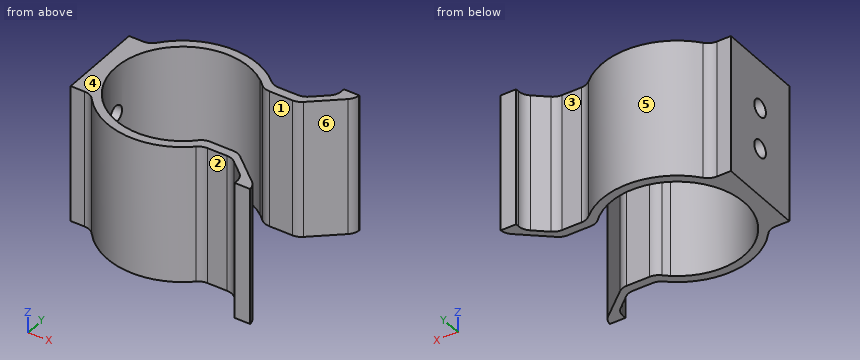
from build123d import *

# Parameters (mm, degrees)
F1_DEPTH = 50.8
F2_R     = 3.175
F3_DEPTH = 127
F5_DEPTH = 50.8
F6_DEPTH = 279.4
F7_R     = 5.08


with BuildPart() as f1:
    # F0 (on Top) → F1 (new body)
    with BuildSketch(Plane.XY):
        with BuildLine():
            ThreePointArc((20.2399183732, 19.2610826343), (21.625356316, 17.6914545532), (22.8893718502, 16.0224922001))
            Line((22.8893718502, 16.0224922001), (31.4840450883, 16.0224922001))
            Line((31.4840450883, 16.0224922001), (44.7927798103, 27.3874809633))
            Line((44.7927798103, 27.3874809633), (45.0897253182, 29.6793562902))
            Line((45.0897253182, 29.6793562902), (39.3924824893, 29.6793562902))
            Line((39.3924824893, 29.6793562902), (39.3924824893, 26.1115133762))
            Line((39.3924824893, 26.1115133762), (31.3704274416, 19.2610826343))
            Line((31.3704274416, 19.2610826343), (20.2399183732, 19.2610826343))
        make_face()
        with BuildLine():
            Line((31.4840450883, -16.0224922001), (22.8893718502, -16.0224922001))
            ThreePointArc((22.8893718502, -16.0224922001), (21.625356316, -17.6914545532), (20.2399183732, -19.2610826343))
            Line((20.2399183732, -19.2610826343), (31.3704274416, -19.2610826343))
            Line((31.3704274416, -19.2610826343), (39.3924824893, -26.1115133762))
            Line((39.3924824893, -26.1115133762), (39.3924824893, -29.6793562902))
            Line((39.3924824893, -29.6793562902), (45.0897253182, -29.6793562902))
            Line((45.0897253182, -29.6793562902), (44.7927798103, -27.3874809633))
            Line((44.7927798103, -27.3874809633), (31.4840450883, -16.0224922001))
        make_face()
        with BuildLine():
            ThreePointArc((15.5664999519, -19.2610826343), (-24.765, 0), (15.5664999519, 19.2610826343))
            Line((15.5664999519, 19.2610826343), (20.2399183732, 19.2610826343))
            ThreePointArc((20.2399183732, 19.2610826343), (-27.94, 0), (20.2399183732, -19.2610826343))
            Line((20.2399183732, -19.2610826343), (15.5664999519, -19.2610826343))
        make_face()
        with BuildLine():
            ThreePointArc((15.5664999519, 19.2610826343), (17.3009251144, 17.7195715294), (18.8834575408, 16.0224922001))
            Line((18.8834575408, 16.0224922001), (22.8893718502, 16.0224922001))
            ThreePointArc((22.8893718502, 16.0224922001), (21.625356316, 17.6914545532), (20.2399183732, 19.2610826343))
            Line((20.2399183732, 19.2610826343), (15.5664999519, 19.2610826343))
        make_face()
        with BuildLine():
            Line((22.8893718502, -16.0224922001), (18.8834575408, -16.0224922001))
            ThreePointArc((18.8834575408, -16.0224922001), (17.3009251144, -17.7195715294), (15.5664999519, -19.2610826343))
            Line((15.5664999519, -19.2610826343), (20.2399183732, -19.2610826343))
            ThreePointArc((20.2399183732, -19.2610826343), (21.625356316, -17.6914545532), (22.8893718502, -16.0224922001))
        make_face()
    extrude(amount=F1_DEPTH)

    # F2 (on Right) → F3 (cut)
    with BuildSketch(Plane.YZ):
        with Locations((0, 33.02)):
            Circle(F2_R)
        with Locations((0, 17.78)):
            Circle(F2_R)
    extrude(amount=-F3_DEPTH, mode=Mode.SUBTRACT)

    # F4 (on face) → F5 (join)
    with BuildSketch(Plane.XY.offset(50.8)):
        Polygon((-26.6156196594, 0), (-22.9919110776, 15.875), (-30.6119110776, 15.875), (-30.6119110776, -15.875), (-22.9919110776, -15.875), align=None)
    extrude(amount=-F5_DEPTH)

    # F2 (on Right) → F6 (cut)
    with BuildSketch(Plane.YZ):
        with Locations((0, 33.02)):
            Circle(F2_R)
        with Locations((0, 17.78)):
            Circle(F2_R)
    extrude(amount=-F6_DEPTH, mode=Mode.SUBTRACT)

    # F7
    f7_edges = [f1.edges().sort_by_distance(p)[0] for p in [
        (-22.991911, 15.875, 25.4),
        (-22.991911, -15.875, 25.4),
        (20.239918, -19.261083, 25.4),
        (31.370427, -19.261083, 25.4),
        (39.392482, -26.111513, 25.4),
        (31.484045, -16.022492, 25.4),
        (18.883458, -16.022492, 25.4),
        (44.79278, -27.387481, 25.4),
        (44.79278, 27.387481, 25.4),
        (31.484045, 16.022492, 25.4),
        (31.370427, 19.261083, 25.4),
        (39.392482, 26.111513, 25.4),
        (20.239918, 19.261083, 25.4),
        (18.883458, 16.022492, 25.4),
    ]]
    fillet(f7_edges, radius=F7_R)


solid = f1.part
Geometry check sheet. Reference: the model listing, model coordinates, mm. Face numbers are marked on the shaded views. A direction names the side the tool comes from. Give positions to 0.01 mm unless a question says otherwise; leave off trailing zeros. Write each loop counter-clockwise with the first axis right and the second up, starting at its lowest first coordinate (ties: lowest second). Pieces come first, ordered by that corner, then holes. Notation, with made-up numbers: M 58.5,-2.75 L 64.5,-2.75 A23 cw 64.5,20.25 Z; hole C 56.5,-24.75 d4. An arc over 180 degrees is marked long. One line per question, with ' | ' between items.
1. Scan lines: line 1 along Z through (x, y) = (-26, 0) (3 decimals); line 2 along Y through (x, z) = (0, 28) (3 decimals); line 3 along Y through (x, z) = (-28.5, 17.78) (3 decimals). Record each from-to range of solid material in increasing order. Write a range as from..to.
Ans:
line 1: 0..14.605, 20.955..29.845, 36.195..50.8 | line 2: -27.94..-24.765, 24.765..27.94 | line 3: -15.875..-3.175, 3.175..15.875
2. Cross-section at B-B (x = 0). Enter the section's corners in (y, z) (3 decimals), plus the area to 3 significant figures.
Ans:
outline: M -27.94,0 L -24.765,0 L -24.765,50.8 L -27.94,50.8 Z; M 24.765,0 L 27.94,0 L 27.94,50.8 L 24.765,50.8 Z | area: 323 mm2
3. Cross-section at C-C (x = 13). Enter the section's corners in (y, z), plus the area to 3 significant figures.
Ans:
outline: M -24.73,0 L -21.08,0 L -21.08,50.8 L -24.73,50.8 Z; M 21.08,0 L 24.73,0 L 24.73,50.8 L 21.08,50.8 Z | area: 371 mm2
4. Gauge pin test, flat ends, axial feed: pin 1 (9.5 mm diameter, centred on x = 26.5, z = 21, fed in from +Y); pin 2 (5.5 mm diameter, centred on x = -27.5, z = 30.5, fed in from -Y); pin 3 (1 mm diameter, centred on y = -29, z = 24.5, fed in from -X); pin 4 (5 mm diameter, centred on y = 0, z = 33.02, fed in from -X). Record the tip position at first contact, or that the pin passes through.
Ans:
pin 1: y = 19.57 | pin 2: y = -15.93 | pin 3: x = 39.39 | pin 4: through
5. Cross-section at A-A (y = 0). Enter the section's corners in (x, z) (3 decimals).
Ans:
outline: M -30.612,0 L -24.765,0 L -24.765,14.605 L -30.612,14.605 Z; M -30.612,20.955 L -24.765,20.955 L -24.765,29.845 L -30.612,29.845 Z; M -30.612,36.195 L -24.765,36.195 L -24.765,50.8 L -30.612,50.8 Z
6. Mould release check, pull along X, two halves, no side actions. Record for the marked faces 4, 5 and 6: released by +X, released by -X, zero draft, split by the parting line, or undercut.
Ans:
face 4: zero draft | face 5: undercut | face 6: released by +X
7. Set-up check for the marked faces 1, 2 and 3: record each of +Z, -Z, +X, -X, +Y, -Y from which the full face is reachable in a straight line by a thin tool's end or side.
Ans:
face 1: +Z, -Z, +X | face 2: +Z, -Z, -Y | face 3: +Z, -Z, +Y
8. Cross-section at D-D (y = -11.5). Enter the section's corners in (x, z).
Ans:
outline: M -30.61,0 L -21.93,0 L -21.93,50.8 L -30.61,50.8 Z
